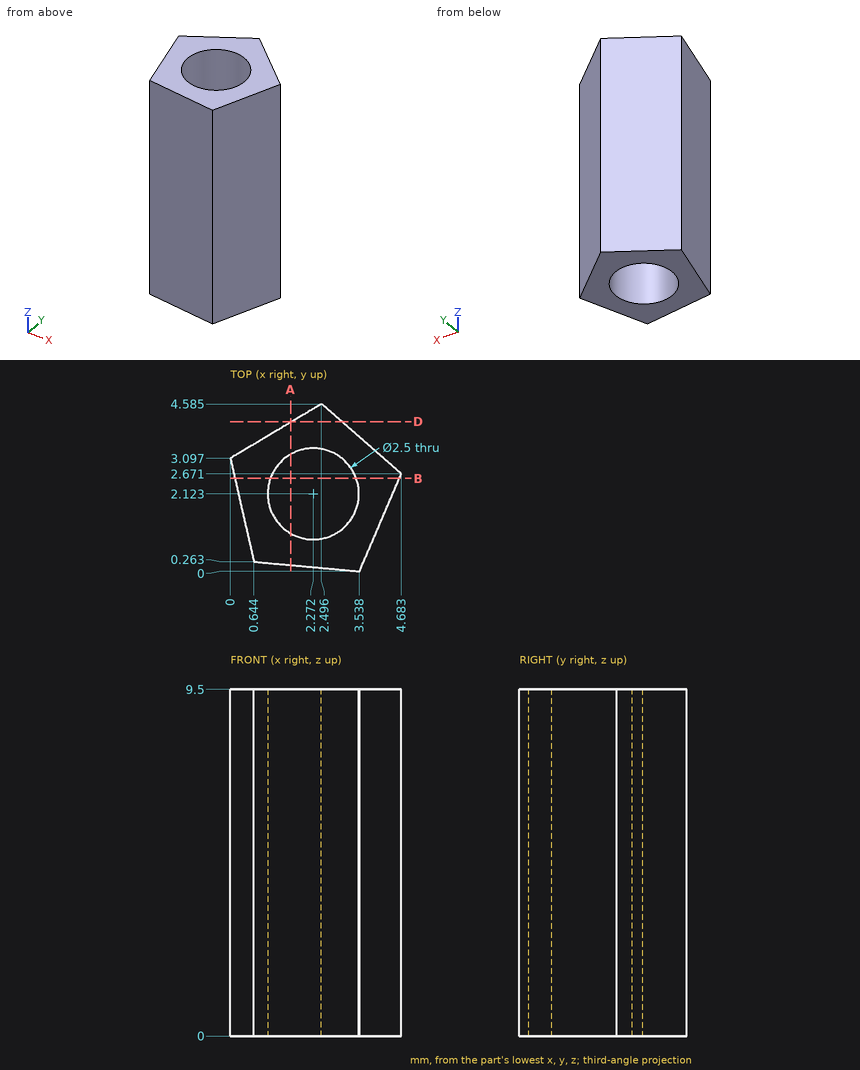
Geometry check sheet. Reference: drawing and pictorial views, mm from the part's lowest x, y, z. Round coordinates to 2 decimals unless told otherwise and drop trailing zeros. Write each loop counter-clockwise with the first axis right and the second up, starting at its lowest first coordinate (ties: lowest second). Pieces come first, ordered by that corner, then holes. Notation, with made-up numbers: (11.5, -16) -> (55.5, -16) arc R26 cw to (55.5, -1) -> close; hole circle Ø11 at (1, 79). An arc over 180 degrees is marked (long way). One line per question, with ' | ' between items. Start each with the question number.
1. Scan lines: line 1 along Y through (x, z) = (2.05, 2) (1 decimal); line 2 along X through (y, z) = (2.3, 1.5) (1 decimal); line 3 along X through (y, z) = (1.95, 4) (1 decimal). Record each from-to range of solid material in increasing order. Write a range as from..to.
2. Sectioned sample at A-A, the plane x = 1.65. Record the cut outline in (y, z).
3. Sectioned sample at D-D, the plane y = 4.1. Record the cut outline in (x, z), then the cut area to 3 significant figures.
4. Sectioned sample at B-B, the plane y = 2.55. Record the cut outline in (x, z) (1 decimal).
Taken from the geometry:
1) line 1: y = 0.1..0.9, 3.4..4.3 | line 2: x = 0.2..1, 3.5..4.5 | line 3: x = 0.3..1, 3.5..4.4
2) outline: (0.17, 0) -> (1.04, 0) -> (1.04, 9.5) -> (0.17, 9.5) -> close; (3.21, 0) -> (4.08, 0) -> (4.08, 9.5) -> (3.21, 9.5) -> close
3) outline: (1.68, 0) -> (3.05, 0) -> (3.05, 9.5) -> (1.68, 9.5) -> close | area: 13.0 mm^2
4) outline: (0.1, 0) -> (1.1, 0) -> (1.1, 9.5) -> (0.1, 9.5) -> close; (3.4, 0) -> (4.6, 0) -> (4.6, 9.5) -> (3.4, 9.5) -> close
